The listing builds one solid part. Answer for the finished solid, in the listing's coordinates (mm). A direction names the side the tool comes from. Round coordinates to 2 decimals unless told otherwise and drop trailing zeros. Order: outer loops, then holes, each group sorted by start corner. A loop starts at its lowest first (then second) coordinate and runs counter-clockwise, first axis right, second up. Notation, with made-up numbers: (68, -6) - (123, -6) arc R20 ccw to (123, 22) - close; hole circle Ø3 at (52.5, 64). An arc over 180 degrees is marked (long way). Write item = value, one per line.
from build123d import *

# Parameters (mm, degrees)
SKETCH1_R           = 7.5
BOSS_EXTRUDE1_DEPTH = 7
CHAMFER1_SIZE       = 1


with BuildPart() as part:
    # Sketch1 → Boss-Extrude1 (new body)
    with BuildSketch(Plane.XY):
        with BuildLine():
            Line((11.5, -2), (11.5, 2))
            Line((11.5, 2), (13.351029923, 2))
            ThreePointArc((13.351029923, 2), (9.545941546, 9.545941546), (2, 13.351029923))
            Line((2, 13.351029923), (2, 11.5))
            Line((2, 11.5), (-2, 11.5))
            Line((-2, 11.5), (-2, 13.351029923))
            ThreePointArc((-2, 13.351029923), (-9.545941546, 9.545941546), (-13.351029923, 2))
            Line((-13.351029923, 2), (-11.5, 2))
            Line((-11.5, 2), (-11.5, -2))
            Line((-11.5, -2), (-13.351029923, -2))
            ThreePointArc((-13.351029923, -2), (-9.545941546, -9.545941546), (-2, -13.351029923))
            Line((-2, -13.351029923), (-2, -11.5))
            Line((-2, -11.5), (2, -11.5))
            Line((2, -11.5), (2, -13.351029923))
            ThreePointArc((2, -13.351029923), (9.545941546, -9.545941546), (13.351029923, -2))
            Line((13.351029923, -2), (11.5, -2))
        make_face()
        Circle(SKETCH1_R, mode=Mode.SUBTRACT)
    extrude(amount=BOSS_EXTRUDE1_DEPTH)

    # Chamfer1
    chamfer1_edges = [part.edges().sort_by_distance(p)[0] for p in [
        (12.425514961, 2, 7),
        (9.545941546, 9.545941546, 7),
        (2, 12.425514961, 7),
        (0, 11.5, 7),
        (-2, 12.425514961, 7),
        (-9.545941546, 9.545941546, 7),
        (-12.425514961, 2, 7),
        (-11.5, 0, 7),
        (-12.425514961, -2, 7),
        (-9.545941546, -9.545941546, 7),
        (-2, -12.425514961, 7),
        (0, -11.5, 7),
        (2, -12.425514961, 7),
        (9.545941546, -9.545941546, 7),
        (12.425514961, -2, 7),
        (11.5, 0, 7),
    ]]
    chamfer(chamfer1_edges, length=CHAMFER1_SIZE)


solid = part.part
Q1. Section C-C on z = 2.75 is taken. Determine the outline of the cut face in (x, y).
Model answer:
outline = (-13.35, -2) arc R13.5 ccw to (-2, -13.35) - (-2, -11.5) - (2, -11.5) - (2, -13.35) arc R13.5 ccw to (13.35, -2) - (11.5, -2) - (11.5, 2) - (13.35, 2) arc R13.5 ccw to (2, 13.35) - (2, 11.5) - (-2, 11.5) - (-2, 13.35) arc R13.5 ccw to (-13.35, 2) - (-11.5, 2) - (-11.5, -2) - close; hole circle Ø15 at (0, 0)
Q2. Find the intervals of material crossed by line 1 (Y direction, x = 0, z = 5); line 2 (Y direction, x = 6.5, z = 1.5); line 3 (X direction, y = 1.75, z = 3), in increasing order. Write a range as from..to.
Model answer:
line_1 = -11.5..-7.5, 7.5..11.5
line_2 = -11.83..-3.74, 3.74..11.83
line_3 = -11.5..-7.29, 7.29..11.5
Q3. For faces 4 (the face through (-12, 2, 3)), 5 (the face through (0, 11, 6.5)), 6 (the face through (11.5, 0, 3)), determine the directions among +Z, -Z, +X, -X, +Y, -Y from which every point of the face is accessible in a straight line to the end or side of a thin tool.
Model answer:
face_4 = +Z, -Z, -X
face_5 = +Z, +Y
face_6 = +Z, -Z, +X
Q4. Determine the mould class of faces 1 (the face through (-7.493, 0.33, 3.451)), 2 (the face through (-9.03, -8.87, 6.84)), 3 (the face through (-8.87, 9.03, 6.84)) for opening direction Y: released by +Y, released by -Y, zero draft, split by the parting line, or undercut.
Model answer:
face_1 = undercut
face_2 = released by -Y
face_3 = released by +Y
Q5. Flat-ended cylindrical pins translate along their axes: P1, Ø0.9, axis at y = -12, z = 2, coming from the +X side; P2, Ø2, axis at y = 3.5, z = 5, coming from the -X side; P3, Ø8, axis at x = -2, y = -5.5, coming from the -Z side; P4, Ø0.6, axis at x = -12.5, z = 3, coming from the +Y side. Find the tip coordinate at first contact, or state that the pin passes through.
Model answer:
P1 = 6.99
P2 = -13.27
P3 = 0
P4 = 5.78
Q6. Section A-A on x = 0 is taken. Determine the outline of the cut face in (y, z), then the cut area to 3 significant figures.
Model answer:
outline = (-11.5, 0) - (-7.5, 0) - (-7.5, 7) - (-10.5, 7) - (-11.5, 6) - close; (7.5, 0) - (11.5, 0) - (11.5, 6) - (10.5, 7) - (7.5, 7) - close
area = 55.0 mm^2
